Work out the finished part from the listing and answer in its coordinate system (mm). A direction names the side the tool comes from. Round coordinates to 2 decimals unless told otherwise and drop trailing zeros. Order: outer loops, then holes, each group sorted by start corner. A loop starts at its lowest first (then second) coordinate and runs counter-clockwise, first axis right, second up. Notation, with made-up numbers: (4.25, 64) -> (36.25, 64) arc R18 ccw to (36.25, 77) -> close; hole circle Ø9 at (22.5, -23). An arc over 180 degrees is marked (long way). Use a Markdown table: item, result. Add a question column.
Item 1: Flat-ended cylindrical pins translate along their axes: P1, Ø8, axis at y = 7, z = -3, coming from the +X side; P2, Ø20, axis at x = -31, z = 3.5, coming from the +Y side; P3, Ø12, axis at x = -8.5, z = -9, coming from the +Y side; P4, Ø2.5, axis at y = 10, z = -18, coming from the -X side. Find the tip coordinate at first contact, or state that the pin passes through.
Item 2: A tool of negligible diameter and unlimited length cuts with its end or side. For faces 1 (the flat face through (-32.45, 9, 26)), 2 (the flat face through (30.45, 10, -26)), 3 (the flat face through (-1, 5, 0)), 4 (the flat face through (32.45, 9, -26)), 5 (the flat face through (50.1, 5.5, 6)), from which of +Z, -Z, +X, -X, +Y, -Y can it reach the whole face along a straight path? Write none if from no direction.
Item 3: A cutting plane is placed at B-B, the plane x = -35.45. Give the number of separate pieces and of enclosed holes in the cut face, plus the area to 3 significant figures.
Item 4: Find the intervals of material crossed by L1, parallel to X at y = 7.25, z = 0; L2, parallel to X at y = 5.5, z = -26; L3, parallel to X at y = 4.25, z = 26, in increasing order. Write a range as [from, to].
Item 5: For a pull along Z with two mould halves and no side action, classify faces 6 (the flat face through (-37, 10.8, 27)), 7 (the flat face through (1, 4, -30)), 8 (the cylindrical face through (-25.328, 11.655, 8.078)) as +Z half, -Z half, draft (parallel to the pull), parting line (faces both ways), or undercut.
Item 6: A cutting plane is placed at A-A, the plane z = 14.5. Determine the outline of the cut face in (x, y).
Item 7: A cutting plane is placed at D-D, the plane x = -6. Determine the outline of the cut face in (y, z).
from build123d import *

# Parameters (mm, degrees)
SKETCH1_W                 = 119.1
SKETCH1_H                 = 60
BOSS_EXTRUDE1_DEPTH       = 5
BOSS_EXTRUDE2_DEPTH       = 24
MIRROR2_COPY_1_DEPTH      = 24
SKETCH3_R                 = 1.75
CUT_EXTRUDE1_DEPTH        = 102.850411143
MIRROR4_COPY_1_SKETCH_R   = 1.75
MIRROR4_COPY_1_DEPTH      = 102.850411143
MIRROR5_COPY_1_SKETCH_R   = 1.75
MIRROR5_COPY_1_DEPTH      = 102.850411143
MIRROR5_COPY_2_SKETCH_R   = 1.75
MIRROR5_COPY_2_DEPTH      = 102.850411143
MIRROR5_COPY_3_SKETCH_R   = 1.75
MIRROR5_COPY_3_DEPTH      = 102.850411143
SKETCH4_R                 = 8
SKETCH4_R_2               = 4
BOSS_EXTRUDE3_DEPTH       = 8.4
CUT_EXTRUDE3_DEPTH        = 6
SKETCH7_R                 = 1.561398203
CUT_EXTRUDE4_DEPTH        = 8
SKETCH8_R                 = 4
CUT_EXTRUDE5_DEPTH        = 8
SKETCH9_W                 = 10
SKETCH9_H                 = 9.8
SKETCH9_W_2               = 6
SKETCH9_H_2               = 2.8
BOSS_EXTRUDE4_DEPTH       = 8
MIRROR9_COPY_1_SKETCH_W   = 10
MIRROR9_COPY_1_SKETCH_H   = 9.8
MIRROR9_COPY_1_SKETCH_W_2 = 6
MIRROR9_COPY_1_SKETCH_H_2 = 2.8
MIRROR9_COPY_1_DEPTH      = 8
SKETCH10_R                = 1.55
CUT_EXTRUDE6_DEPTH        = 69.3025805


with BuildPart() as part:
    # Sketch1 → Boss-Extrude1 (new body)
    with BuildSketch(Plane(origin=(0, 0, 0), x_dir=(1, 0, 0), z_dir=(0, 1, 0))):
        Rectangle(SKETCH1_W, SKETCH1_H)
    extrude(amount=BOSS_EXTRUDE1_DEPTH)

    # Sketch2 → Boss-Extrude2 (add)
    with BuildSketch(Plane.XY.offset(30)):
        with BuildLine():
            Line((-59.55, 13.55), (-59.55, 5))
            Line((-59.55, 5), (-40.45, 5))
            Line((-40.45, 5), (-40.45, 13.55))
            Line((-40.45, 13.55), (-42.45, 13.55))
            ThreePointArc((-42.45, 13.55), (-50, 6), (-57.55, 13.55))
            Line((-57.55, 13.55), (-59.55, 13.55))
        make_face()
    boss_extrude2 = extrude(amount=-BOSS_EXTRUDE2_DEPTH)

    # Mirror1: Boss-Extrude2 across plane
    add(boss_extrude2.mirror(Plane.XY))

    # Mirror2: Boss-Extrude2 across plane
    add(boss_extrude2.mirror(Plane(origin=(0, 0, 0), x_dir=(0, 0, 1), z_dir=(1, 0, 0))))

    # Mirror2 copy 1 sketch → Mirror2 copy 1 (add)
    with BuildSketch(Plane(origin=(0, 0, -30), x_dir=(-1, 0, 0), z_dir=(0, 0, -1))):
        with BuildLine():
            Line((-59.55, 13.55), (-59.55, 5))
            Line((-59.55, 5), (-40.45, 5))
            Line((-40.45, 5), (-40.45, 13.55))
            Line((-40.45, 13.55), (-42.45, 13.55))
            ThreePointArc((-42.45, 13.55), (-50, 6), (-57.55, 13.55))
            Line((-57.55, 13.55), (-59.55, 13.55))
        make_face()
    extrude(amount=-MIRROR2_COPY_1_DEPTH)

    # Sketch3 → Cut-Extrude1 (cut, symmetric)
    with BuildSketch(Plane(origin=(-32.275, 32.275, 0), x_dir=(0.7071067811865477, 0.7071067811865475, 0), z_dir=(-0.7071067811865475, 0.7071067811865477, 0))):
        with Locations(Location((-35.355339059, -18, 0), (0, 0, 180))):
            Circle(SKETCH3_R)
    cut_extrude1 = extrude(amount=CUT_EXTRUDE1_DEPTH, both=True, mode=Mode.SUBTRACT)

    # Mirror3: Cut-Extrude1 across plane
    add(cut_extrude1.mirror(Plane.ZY.offset(50)), mode=Mode.SUBTRACT)

    # Mirror4: Cut-Extrude1 across plane
    add(cut_extrude1.mirror(Plane.XY), mode=Mode.SUBTRACT)

    # Mirror4 copy 1 sketch → Mirror4 copy 1 (cut, symmetric)
    with BuildSketch(Plane(origin=(-67.725, 32.275, 0), x_dir=(-0.7071067811865477, 0.7071067811865475, 0), z_dir=(0.7071067811865475, 0.7071067811865477, 0))):
        with Locations(Location((-35.355339059, -18, 0), (0, 0, 180))):
            Circle(MIRROR4_COPY_1_SKETCH_R)
    extrude(amount=MIRROR4_COPY_1_DEPTH, both=True, mode=Mode.SUBTRACT)

    # Mirror5: Cut-Extrude1 across plane
    add(cut_extrude1.mirror(Plane(origin=(0, 0, 0), x_dir=(0, 0, 1), z_dir=(1, 0, 0))), mode=Mode.SUBTRACT)

    # Mirror5 copy 1 sketch → Mirror5 copy 1 (cut, symmetric)
    with BuildSketch(Plane(origin=(67.725, 32.275, 0), x_dir=(0.7071067811865477, 0.7071067811865475, 0), z_dir=(-0.7071067811865475, 0.7071067811865477, 0))):
        with Locations(Location((-35.355339059, -18, 0), (0, 0, 180))):
            Circle(MIRROR5_COPY_1_SKETCH_R)
    extrude(amount=MIRROR5_COPY_1_DEPTH, both=True, mode=Mode.SUBTRACT)

    # Mirror5 copy 2 sketch → Mirror5 copy 2 (cut, symmetric)
    with BuildSketch(Plane(origin=(32.275, 32.275, 0), x_dir=(-0.7071067811865477, 0.7071067811865475, 0), z_dir=(0.7071067811865475, 0.7071067811865477, 0))):
        with Locations(Location((-35.355339059, -18, 0), (0, 0, 180))):
            Circle(MIRROR5_COPY_2_SKETCH_R)
    extrude(amount=MIRROR5_COPY_2_DEPTH, both=True, mode=Mode.SUBTRACT)

    # Mirror5 copy 3 sketch → Mirror5 copy 3 (cut, symmetric)
    with BuildSketch(Plane(origin=(67.725, 32.275, 0), x_dir=(0.7071067811865477, 0.7071067811865475, 0), z_dir=(-0.7071067811865475, 0.7071067811865477, 0))):
        with Locations((-35.355339059, 18)):
            Circle(MIRROR5_COPY_3_SKETCH_R)
    extrude(amount=MIRROR5_COPY_3_DEPTH, both=True, mode=Mode.SUBTRACT)

    # Sketch4 → Boss-Extrude3 (add)
    with BuildSketch(Plane(origin=(0, 5, 0), x_dir=(1, 0, 0), z_dir=(0, 1, 0))):
        with Locations((-30, 0)):
            Circle(SKETCH4_R)
        with Locations(Location((-30, 0, 0), (0, 0, 270))):
            Circle(SKETCH4_R_2, mode=Mode.SUBTRACT)
        with BuildLine():
            Line((-30.217325584, -7.997047555), (-27.950944845, -10.99096779))
            Line((-27.950944845, -10.99096779), (-19.977792674, -4.95533655))
            Line((-19.977792674, -4.95533655), (-22.244173413, -1.961416314))
            ThreePointArc((-22.244173413, -1.961416314), (-25.171495008, -6.378521736), (-30.217325584, -7.997047555))
        make_face()
    boss_extrude3 = extrude(amount=BOSS_EXTRUDE3_DEPTH)

    # Sketch6 → Cut-Extrude3 (cut)
    with BuildSketch(Plane(origin=(0, 13.4, 0), x_dir=(1, 0, 0), z_dir=(0, 1, 0))):
        Polygon((-28.951635844, -6.355386109), (-24.167744542, -2.734007365), (-22.477767795, -4.966489973), (-27.261659097, -8.587868717), align=None)
    cut_extrude3 = extrude(amount=-CUT_EXTRUDE3_DEPTH, mode=Mode.SUBTRACT)

    # Sketch7 → Cut-Extrude4 (cut)
    with BuildSketch(Plane(origin=(-4.893022101, 0, -6.463749727), x_dir=(0.797315217025082, 0, -0.6035631240394382), z_dir=(0.6035631240394382, 0, 0.797315217025082))):
        with Locations((-23.919456511, 10.6)):
            Circle(SKETCH7_R)
    cut_extrude4 = extrude(amount=-CUT_EXTRUDE4_DEPTH, mode=Mode.SUBTRACT)

    # Mirror7: Boss-Extrude3, Cut-Extrude3, Cut-Extrude4 across plane
    add(boss_extrude3.mirror(Plane(origin=(0, 0, 0), x_dir=(0, 0, 1), z_dir=(1, 0, 0))))
    add(cut_extrude3.mirror(Plane(origin=(0, 0, 0), x_dir=(0, 0, 1), z_dir=(1, 0, 0))), mode=Mode.SUBTRACT)
    add(cut_extrude4.mirror(Plane(origin=(0, 0, 0), x_dir=(0, 0, 1), z_dir=(1, 0, 0))), mode=Mode.SUBTRACT)

    # Sketch8 → Cut-Extrude5 (cut)
    with BuildSketch(Plane(origin=(0, 5, 0), x_dir=(1, 0, 0), z_dir=(0, 1, 0))):
        with Locations(Location((-30, 0, 0), (0, 0, 270))):
            Circle(SKETCH8_R)
        with Locations(Location((30, 0, 0), (0, 0, 270))):
            Circle(SKETCH8_R)
    extrude(amount=-CUT_EXTRUDE5_DEPTH, mode=Mode.SUBTRACT)

    # Sketch9 → Boss-Extrude4 (add)
    with BuildSketch(Plane.XY.offset(30)):
        with Locations((-35.45, 9.9)):
            Rectangle(SKETCH9_W, SKETCH9_H)
        with Locations((-35.45, 9.4)):
            Rectangle(SKETCH9_W_2, SKETCH9_H_2, mode=Mode.SUBTRACT)
    boss_extrude4 = extrude(amount=-BOSS_EXTRUDE4_DEPTH)

    # Mirror8: Boss-Extrude4 across plane
    add(boss_extrude4.mirror(Plane(origin=(0, 0, 0), x_dir=(0, 0, 1), z_dir=(1, 0, 0))))

    # Mirror9: Boss-Extrude4 across plane
    add(boss_extrude4.mirror(Plane.XY))

    # Mirror9 copy 1 sketch → Mirror9 copy 1 (add)
    with BuildSketch(Plane(origin=(0, 0, -30), x_dir=(-1, 0, 0), z_dir=(0, 0, -1))):
        with Locations((-35.45, 9.9)):
            Rectangle(MIRROR9_COPY_1_SKETCH_W, MIRROR9_COPY_1_SKETCH_H)
        with Locations((-35.45, 9.4)):
            Rectangle(MIRROR9_COPY_1_SKETCH_W_2, MIRROR9_COPY_1_SKETCH_H_2, mode=Mode.SUBTRACT)
    extrude(amount=-MIRROR9_COPY_1_DEPTH)

    # Sketch10 → Cut-Extrude6 (cut, through all)
    with BuildSketch(Plane(origin=(0, 14.8, 0), x_dir=(1, 0, 0), z_dir=(0, 1, 0))):
        with Locations(Location((-35.45, 26, 0), (0, 0, 270))):
            Circle(SKETCH10_R)
        with Locations(Location((35.45, 26, 0), (0, 0, 270))):
            Circle(SKETCH10_R)
        with Locations(Location((35.45, -26, 0), (0, 0, 270))):
            Circle(SKETCH10_R)
        with Locations(Location((-35.45, -26, 0), (0, 0, 270))):
            Circle(SKETCH10_R)
    extrude(amount=-CUT_EXTRUDE6_DEPTH, mode=Mode.SUBTRACT)


solid = part.part
Reported:
| question | item | result |
|---|---|---|
| 1 | P1 | x = 59.55 |
| 1 | P2 | y = 13.55 |
| 1 | P3 | y = 5 |
| 1 | P4 | x = -58.78 |
| 2 | face 1 | +Z |
| 2 | face 2 | -Z, +Y |
| 2 | face 3 | +Y |
| 2 | face 4 | -Z |
| 2 | face 5 | +X, +Y |
| 3 | separate pieces | 7 |
| 3 | enclosed holes | 0 |
| 3 | area | 436 mm² |
| 4 | L1 | [-38, -34], [-26, -22], [22, 26], [34, 38] |
| 4 | L2 | [-59.55, -37], [-33.9, -30.45], [30.45, 33.9], [37, 59.55] |
| 4 | L3 | [-59.55, -37], [-33.9, 33.9], [37, 59.55] |
| 5 | face 6 | draft |
| 5 | face 7 | -Z half |
| 5 | face 8 | undercut |
| 6 | outline | (-59.55, 0) -> (59.55, 0) -> (59.55, 13.55) -> (57.55, 13.55) arc R7.55 cw to (42.45, 13.55) -> (40.45, 13.55) -> (40.45, 5) -> (-40.45, 5) -> (-40.45, 13.55) -> (-42.45, 13.55) arc R7.55 cw to (-57.55, 13.55) -> (-59.55, 13.55) -> close |
| 7 | outline | (0, -30) -> (5, -30) -> (5, 30) -> (0, 30) -> close |
